Verification items for the finished model (mm, model axes). Face numbers are marked on the shaded views. A direction names the side the tool comes from. Give positions to 0.01 mm unless a question says otherwise; leave off trailing zeros. Order: outer loops, then holes, each group sorted by start corner. A loop starts at its lowest first (then second) coordinate and runs counter-clockwise, first axis right, second up. Notation, with made-up numbers: (0.25, -38.5) -> (55.25, -38.5) arc R20 ccw to (55.25, -10.5) -> close; hole circle Ø3 at (-28.75, 36). An arc over 180 degrees is marked (long way). Return JSON: item names as keys, results as strings. Group by question number.
(1) Cross-section at B-B on z = -1.15. Enter the section's corners in (x, y) (1 decimal).
(2) Thickness scan on line 1 along Y through (x, z) = (-9, -2.15); line 2 along Y through (x, z) = (4, 2.15); line 3 along X through (y, z) = (-14, -2.05). Record the ranges inside material, lowest first.
(3) Tool access check on the marked faces 1 and 2. Record the directions out of +Z, -Z, +X, -X, +Y, -Y that give a thin tool (end or side, any length) a straight path to the whole face; none if there is none.
(4) Cross-section at C-C on x = 4. Enter the section's corners in (y, z).
(5) Depth check by flat-ended pin: pin 1 Ø3 at (y, z) = (7, -0.5) entering from +X; pin 2 Ø1.8 at (y, z) = (0, 0.5) entering from +X; pin 3 Ø1.5 at (x, z) = (16.5, 2) entering from +Y. Enter the tip coordinate at first touch or a pass-through.
(6) Release check for a two-part mould opening along Y. For the marked faces 3, 4 and 5 record: pulls with the +Y half, pulls with the -Y half, needs draft (parallel to the pull), parting line crosses it, or undercut.
(7) Cross-section at D-D on x = -31.5. Enter the section's corners in (y, z).
(8) Cross-section at A-A on y = 9. Enter the section's corners in (x, z), then the cut area to 3 significant figures.
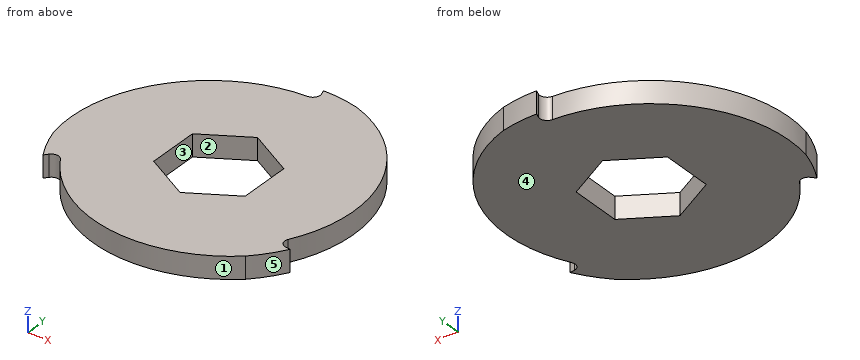
from build123d import *

# Parameters (mm, degrees)
BOSS_EXTRUDE1_DEPTH = 3
FILLET1_R           = 2


with BuildPart() as part:
    # Sketch1 → Boss-Extrude1 (new, symmetric)
    with BuildSketch(Plane.XY):
        with BuildLine():
            ThreePointArc((10.093942759, 37.671107225), (5.090521497, 38.666349594), (0, 39))
            Line((0, 39), (1.467076979, 34.969239127))
            ThreePointArc((1.467076979, 34.969239127), (-29.031358559, 21.929979589), (-37.671107225, -10.093942759))
            ThreePointArc((-37.671107225, -10.093942759), (-36.031301768, -14.924653862), (-33.774990748, -19.5))
            Line((-33.774990748, -19.5), (-31.017787925, -16.21409363))
            ThreePointArc((-31.017787925, -16.21409363), (-4.476240149, -36.106883814), (27.577164466, -27.577164466))
            ThreePointArc((27.577164466, -27.577164466), (30.940780271, -23.741695731), (33.774990748, -19.5))
            Line((33.774990748, -19.5), (29.550710946, -18.755145497))
            ThreePointArc((29.550710946, -18.755145497), (33.507598709, 14.176904224), (10.093942759, 37.671107225))
        make_face()
        Polygon((-12.5, 7.216878365), (0, 14.43375673), (12.5, 7.216878365), (12.5, -7.216878365), (0, -14.43375673), (-12.5, -7.216878365), align=None, mode=Mode.SUBTRACT)
    extrude(amount=BOSS_EXTRUDE1_DEPTH, both=True)

    # Fillet1
    fillet1_edges = [part.edges().sort_by_distance(p)[0] for p in [
        (1.467076979, 34.969239127, 0),
        (29.550710946, -18.755145497, 0),
        (-31.017787925, -16.21409363, 0),
    ]]
    fillet(fillet1_edges, radius=FILLET1_R)


solid = part.part
Verdict:
{
 "1": {"outline": "(-37.7, -10.1) arc R39 ccw to (-33.8, -19.5) -> (-32.9, -18.4) arc R2 cw to (-29.6, -18.7) arc R38 ccw to (27.6, -27.6) arc R39 ccw to (33.8, -19.5) -> (32.4, -19.3) arc R2 cw to (31, -16.3) arc R38 ccw to (10.1, 37.7) arc R39 ccw to (0, 39) -> (0.5, 37.7) arc R2 cw to (-1.3, 35) arc R38 ccw to start; hole (-12.5, -7.2) -> (0, -14.4) -> (12.5, -7.2) -> (12.5, 7.2) -> (0, 14.4) -> (-12.5, 7.2) -> close"},
 "2": {"line 1": "-34.94 to -9.24, 9.24 to 34.01", "line 2": "-36.78 to -12.12, 12.12 to 38.79", "line 3": "-36.4 to -0.75, 0.75 to 32.15"},
 "3": {"face 1": "+Z, -Z, -Y", "face 2": "+Z, -Z"},
 "4": {"outline": "(-36.78, -3) -> (-12.12, -3) -> (-12.12, 3) -> (-36.78, 3) -> close; (12.12, -3) -> (38.79, -3) -> (38.79, 3) -> (12.12, 3) -> close"},
 "5": {"pin 1": "x = 35.4", "pin 2": "x = 35.57", "pin 3": "y = 35.17"},
 "6": {"face 3": "undercut", "face 4": "needs draft", "face 5": "pulls with the -Y half"},
 "7": {"outline": "(-17.72, -3) -> (18.76, -3) -> (18.76, 3) -> (-17.72, 3) -> close"},
 "8": {"outline": "(-36.4, -3) -> (-9.41, -3) -> (-9.41, 3) -> (-36.4, 3) -> close; (9.41, -3) -> (34.89, -3) -> (34.89, 3) -> (9.41, 3) -> close", "area": "315 mm²"}
}
